```python
from build123d import *

# Parameters (mm, degrees)
CROQUIS1_W               = 15.5
CROQUIS1_H               = 17.5
SALIENTE_EXTRUIR1_DEPTH  = 11.5
CROQUIS2_W               = 12.3
CROQUIS2_H               = 10.05
CORTAR_EXTRUIR1_DEPTH    = 23.328513161
REDONDEO1_R              = 1
CROQUIS3_W               = 9
CROQUIS3_H               = 3
SALIENTE_EXTRUIR4_DEPTH  = 11
CROQUIS12_R              = 1.1
CORTAR_EXTRUIR7_DEPTH    = 23.369063458
CROQUIS13_W              = 18.078388853
CROQUIS13_H              = 17.5
CORTAR_EXTRUIR8_DEPTH    = 24.672241128
REDONDEO1_OF_SIMETR_A2_R = 1
REDONDEO6_R              = 2
CROQUIS15_W              = 6.15
CROQUIS15_H              = 1.2
CROQUIS15_H_2            = 1
CROQUIS15_H_3            = 1.5
CORTAR_EXTRUIR10_DEPTH   = 10.05
CROQUIS17_W              = 2.5
CROQUIS17_H              = 4
SALIENTE_EXTRUIR6_DEPTH  = 2.5
CROQUIS19_R              = 2.5
CORTAR_EXTRUIR12_DEPTH   = 4
CROQUIS20_W              = 2
CROQUIS20_H              = 1.8
CORTAR_EXTRUIR13_DEPTH   = 7.05


with BuildPart() as part:
    # Croquis1 → Saliente-Extruir1 (new body)
    with BuildSketch(Plane(origin=(0, 0, 0), x_dir=(1, 0, 0), z_dir=(0, 1, 0))):
        Rectangle(CROQUIS1_W, CROQUIS1_H)
    saliente_extruir1 = extrude(amount=SALIENTE_EXTRUIR1_DEPTH)

    # Croquis2 → Cortar-Extruir1 (cut, through all)
    with BuildSketch(Plane.XY.offset(8.75)):
        with Locations((0, 5.025)):
            Rectangle(CROQUIS2_W, CROQUIS2_H)
    cortar_extruir1 = extrude(amount=-CORTAR_EXTRUIR1_DEPTH, mode=Mode.SUBTRACT)

    # Redondeo1
    redondeo1_edges = [part.edges().sort_by_distance(p)[0] for p in [
        (7.75, 11.5, 0),
        (-7.75, 11.5, 0),
    ]]
    fillet(redondeo1_edges, radius=REDONDEO1_R)

    # Croquis13 → Cortar-Extruir8 (cut, through all)
    with BuildSketch(Plane(origin=(0, 11.5, 0), x_dir=(1, 0, 0), z_dir=(0, 1, 0))):
        with Locations((-9.039194426, 0)):
            Rectangle(CROQUIS13_W, CROQUIS13_H)
    extrude(amount=-CORTAR_EXTRUIR8_DEPTH, mode=Mode.SUBTRACT)

    # Simetría2: Saliente-Extruir1 across plane
    add(saliente_extruir1.mirror(Plane(origin=(0, 0, -8.75), x_dir=(0, 0, 1), z_dir=(1, 0, 0))))

    # Simetr_a2 2: Cortar-Extruir1 across plane
    add(cortar_extruir1.mirror(Plane(origin=(0, 0, -8.75), x_dir=(0, 0, 1), z_dir=(1, 0, 0))), mode=Mode.SUBTRACT)


with BuildPart() as body_2:
    # Croquis3 → Saliente-Extruir4 (new body)
    with BuildSketch(Plane(origin=(7.75, 0, 0), x_dir=(0, 0, -1), z_dir=(1, 0, 0))):
        with Locations((4.25, 1.5)):
            Rectangle(CROQUIS3_W, CROQUIS3_H)
    saliente_extruir4 = extrude(amount=SALIENTE_EXTRUIR4_DEPTH)

    # Croquis12 → Cortar-Extruir7 (cut, through all)
    with BuildSketch(Plane(origin=(0, 3, 0), x_dir=(1, 0, 0), z_dir=(0, 1, 0))):
        with Locations(Location((13.5, 4.25, 0), (0, 0, 270))):
            Circle(CROQUIS12_R)
    cortar_extruir7 = extrude(amount=-CORTAR_EXTRUIR7_DEPTH, mode=Mode.SUBTRACT)


with BuildPart() as part_1:
    add(part.part)

    # Simetr_a2 3: Saliente-Extruir4 across plane
    add(saliente_extruir4.mirror(Plane(origin=(0, 0, -8.75), x_dir=(0, 0, 1), z_dir=(1, 0, 0))))

    # Simetr_a2 4: Cortar-Extruir7 across plane
    add(cortar_extruir7.mirror(Plane(origin=(0, 0, -8.75), x_dir=(0, 0, 1), z_dir=(1, 0, 0))), mode=Mode.SUBTRACT)

    # Redondeo1 of Simetría2
    redondeo1_of_simetr_a2_edges = [part_1.edges().sort_by_distance(p)[0] for p in [
        (-7.75, 11.5, 0),
        (7.75, 11.5, 0),
    ]]
    fillet(redondeo1_of_simetr_a2_edges, radius=REDONDEO1_OF_SIMETR_A2_R)

    # Combinar3: union body 2
    add(body_2.part)

    # Redondeo6
    redondeo6_edges = [part_1.edges().sort_by_distance(p)[0] for p in [
        (6.15, 10.05, 0),
        (-6.15, 10.05, 0),
    ]]
    fillet(redondeo6_edges, radius=REDONDEO6_R)

    # Croquis15 → Cortar-Extruir10 (cut)
    with BuildSketch(Plane(origin=(0, 0, 0), x_dir=(-1, 0, 0), z_dir=(0, -1, 0))):
        with Locations((-3.075, 0.15)):
            Rectangle(CROQUIS15_W, CROQUIS15_H)
        with Locations((-3.075, -2.75)):
            Rectangle(CROQUIS15_W, CROQUIS15_H_2)
        with Locations((-3.075, -8)):
            Rectangle(CROQUIS15_W, CROQUIS15_H_3)
        Polygon((6.15, 0.75), (0, 0.75), (0, -0.45), (0, -2.25), (0, -3.25), (0, -7.25), (0, -8.75), (6.15, -8.75), align=None)
    extrude(amount=-CORTAR_EXTRUIR10_DEPTH, mode=Mode.SUBTRACT)

    # Croquis17 → Saliente-Extruir6 (add)
    with BuildSketch(Plane.XZ.offset(-10.05)):
        with Locations((-4.9, 5.25)):
            Rectangle(CROQUIS17_W, CROQUIS17_H)
    extrude(amount=SALIENTE_EXTRUIR6_DEPTH)

    # Croquis19 → Cortar-Extruir12 (cut)
    with BuildSketch(Plane.XY.offset(7.25)):
        with Locations((-3.65, 7.55)):
            Circle(CROQUIS19_R)
    extrude(amount=-CORTAR_EXTRUIR12_DEPTH, mode=Mode.SUBTRACT)

    # Croquis20 → Cortar-Extruir13 (cut)
    with BuildSketch(Plane.XZ.offset(-10.05)):
        with Locations((5.15, 1.35)):
            Rectangle(CROQUIS20_W, CROQUIS20_H)
    extrude(amount=CORTAR_EXTRUIR13_DEPTH, mode=Mode.SUBTRACT)


solid = part_1.part
```
Read the model definition and answer for the solid it produces. Units are mm, in the model's axes. A direction names the side the tool comes from. Round coordinates to 2 decimals unless told otherwise and drop trailing zeros. Write each loop counter-clockwise with the first axis right and the second up, starting at its lowest first coordinate (ties: lowest second). Pieces come first, ordered by that corner, then holes. Notation, with made-up numbers: M -13.75,-10.75 L 23.25,-10.75 A9 cw 23.25,1.25 Z; hole C 55,-11.5 d6. An arc over 180 degrees is marked long. One line per item, written item: value.
Q1. For a pull along X with two mould halves and no side action, classify faces 5 (the cylindrical face through (-7.465, 11.199, -0.123)), 6 (the cylindrical face through (-12.426, 1.521, -4.488)), 7 (the flat face through (18.75, 2, -4)), 8 (the cylindrical face through (-5.398, 9.337, 5.278)) as +X half, -X half, draft (parallel to the pull), parting line (faces both ways), or undercut.
Data:
face 5: -X half
face 6: undercut
face 7: +X half
face 8: undercut
Q2. Find section B-B on z = -4.25. Write down the section's boundary in (x, y).
Data:
outline: M -18.75,0 L -14.6,0 L -14.6,3 L -18.75,3 Z; M -12.4,0 L -6.15,0 L -6.15,8.05 A2 cw -4.15,10.05 L 4.15,10.05 A2 cw 6.15,8.05 L 6.15,0 L 12.4,0 L 12.4,3 L 7.75,3 L 7.75,10.5 A1 ccw 6.75,11.5 L -6.75,11.5 A1 ccw -7.75,10.5 L -7.75,3 L -12.4,3 Z; M 14.6,0 L 18.75,0 L 18.75,3 L 14.6,3 Z
Q3. Straight lines are drawn through the part: line 1 (X direction, y = 0.95, z = -4.25); line 2 (Z direction, x = -13.5, y = 1.1); line 3 (X direction, y = 7.5, z = -0.5). For each, find the intervals that lie inside material, in ascending order. Write a range as [from, to].
Data:
line 1: [-18.75, -14.6], [-12.4, -6.15], [6.15, 12.4], [14.6, 18.75]
line 2: [-8.75, -5.35], [-3.15, 0.25]
line 3: [-7.75, -6.15], [6.15, 7.75]
Q4. Flat-ended cylindrical pins translate along their axes: pin 1 Ø3 at (x, y) = (9, 6) entering from +Z; pin 2 Ø5 at (y, z) = (6.5, 0.5) entering from -X; pin 3 Ø3.5 at (x, y) = (13.5, 1.5) entering from +Z; pin 4 Ø7 at (x, z) = (-12.5, -3.5) entering from +Y. Find the tip coordinate at first contact, or state that the pin passes through.
Data:
pin 1: z = 8.75
pin 2: x = -7.75
pin 3: z = 0.25
pin 4: y = 3
Q5. Find section A-A on x = 13.5. Write down the section's boundary in (y, z).
Data:
outline: M 0,-8.75 L 3,-8.75 L 3,-5.35 L 0,-5.35 Z; M 0,-3.15 L 3,-3.15 L 3,0.25 L 0,0.25 Z
Q6. Find section D-D on x = -9.5. Write down the section's boundary in (y, z).
Data:
outline: M 0,-8.75 L 3,-8.75 L 3,0.25 L 0,0.25 Z
Q7. Which of the six approach directions +Z, -Z, +X, -X, +Y, -Y give full straight-line access (tool end or side, diameter ignored) to faces 1 (the cylindrical face through (5.58, 9.45, -4.81)), 2 (the flat face through (13, 1, 0.25)), 3 (the flat face through (5.7, 9.6, -0.75)), 4 (the flat face through (13, 3, -3))?
Data:
face 1: +Z, -Z, -Y
face 2: +Z, +X, +Y, -Y
face 3: -Y
face 4: +Z, -Z, +X, +Y
Q8. Find section C-C on z = 1.25. Write down the section's boundary in (x, y), plus the area to 3 significant figures.
Data:
outline: M -7.75,0 L -6.15,0 L -6.15,10.05 L 6.15,10.05 L 6.15,0 L 7.75,0 L 7.75,10.5 A1 ccw 6.75,11.5 L -6.75,11.5 A1 ccw -7.75,10.5 Z
area: 54.2 mm2
